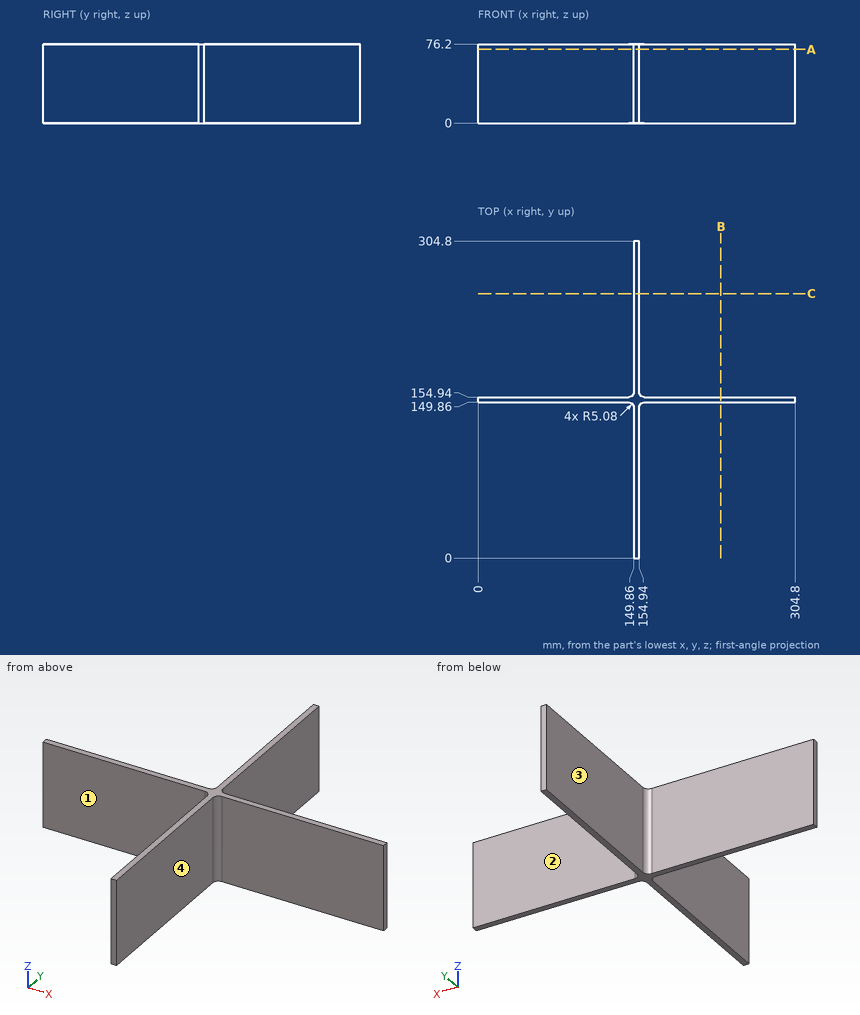
The figure shows three views and two pictorial views of one solid part (mm, origin at its lowest corner). Answer the questions. A direction names the side the tool comes from. Give positions to 0.01 mm unless a question says otherwise; leave off trailing zeros. Write each loop counter-clockwise with the first axis right and the second up, starting at its lowest first coordinate (ties: lowest second). Pieces come first, ordered by that corner, then holes. Notation, with made-up numbers: M 42.5,-34 L 84.5,-34 A26 cw 84.5,3 Z; hole C -38,8 d9. An arc over 180 degrees is marked long. Write each question's results on one line, items separated by ' | '.
Q1. Consider L1, parallel to X at y = 134, z = 66; L2, parallel to X at y = 145.5, z = 4. Determine where each line is inside the solid, lowest interval first. Write a range as from..to.
Output values:
L1: 149.86..154.94 | L2: 149.81..154.99
Q2. Section B-B, the plane x = 233.5 is taken. Write down the section's boundary in (y, z).
Output values:
outline: M 149.86,0 L 154.94,0 L 154.94,76.2 L 149.86,76.2 Z
Q3. Flat-ended cylindrical pins translate along their axes: P1, Ø1, axis at y = 264.5, z = 53.5, coming from the -X side; P2, Ø23, axis at y = 203, z = 51, coming from the +X side; P3, Ø23, axis at x = 53.5, z = 19.5, coming from the +Y side. Find the tip coordinate at first contact, or state that the pin passes through.
Output values:
P1: x = 149.86 | P2: x = 154.94 | P3: y = 154.94
Q4. A tool of negligible diameter and unlimited length cuts with its end or side. For the marked faces 1, 2, 3 and 4, from which of +Z, -Z, +X, -X, +Y, -Y can it reach the whole face along a straight path? Write none if from no direction.
Output values:
face 1: +Z, -Z, -X, -Y | face 2: +Z, -Z, +X, +Y | face 3: +Z, -Z, -X, +Y | face 4: +Z, -Z, +X, -Y
Q5. Section A-A, the plane z = 71 is taken. Write down the section's boundary in (x, y), then the cut area to 3 significant figures.
Output values:
outline: M 0,149.86 L 144.78,149.86 A5.08 cw 149.86,144.78 L 149.86,0 L 154.94,0 L 154.94,144.78 A5.08 cw 160.02,149.86 L 304.8,149.86 L 304.8,154.94 L 160.02,154.94 A5.08 cw 154.94,160.02 L 154.94,304.8 L 149.86,304.8 L 149.86,160.02 A5.08 cw 144.78,154.94 L 0,154.94 Z | area: 3,090 mm2
